Here's how the part is built. I have some questions about the finished solid (model axes, mm). Face numbers are marked on the shaded views. A direction names the side the tool comes from. Round coordinates to 2 decimals unless told otherwise and drop trailing zeros. Order: outer loops, then holes, each group sorted by start corner. A loop starts at its lowest first (then second) coordinate and runs counter-clockwise, first axis right, second up.
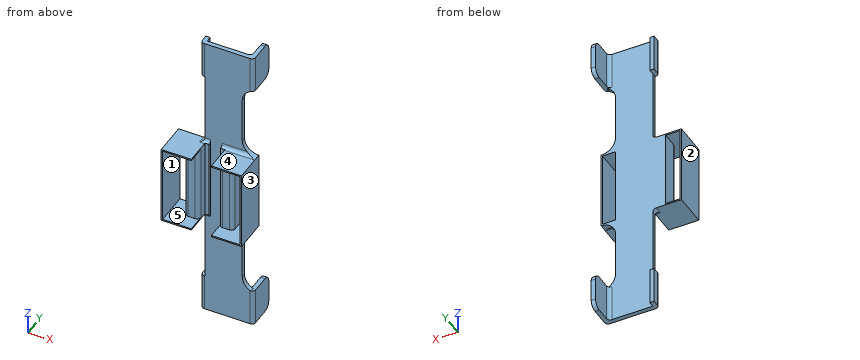
```python
from build123d import *

# Parameters (mm, degrees)
SKETCH1_W                 = 28
SKETCH1_H                 = 28
SKETCH1_W_2               = 27
SKETCH1_H_2               = 27
BOSS_EXTRUDE1_DEPTH       = 5
SKETCH2_W                 = 27
SKETCH2_H                 = 27
BOSS_EXTRUDE2_DEPTH       = 1
SKETCH4_W                 = 7
SKETCH4_H                 = 0.5
CUT_EXTRUDE1_DEPTH        = 4
CUT_EXTRUDE2_DEPTH        = 21.199009877
CUT_EXTRUDE2_DEPTH_BACK   = 21.199009877
SKETCH5_W                 = 5
SKETCH5_H                 = 27
SKETCH7_W                 = 5
SKETCH7_H                 = 27
BOSS_EXTRUDE3_DEPTH       = 4
BOSS_EXTRUDE4_DEPTH       = 5
BOSS_EXTRUDE5_DEPTH       = 5
SKETCH10_W                = 13
SKETCH10_H                = 105
BOSS_EXTRUDE6_DEPTH       = 1.5
SKETCH11_W                = 10
SKETCH11_H                = 28
SKETCH11_W_2              = 5
SKETCH11_H_2              = 27
BOSS_EXTRUDE7_DEPTH       = 1.5
SKETCH12_W                = 3
SKETCH12_H                = 13
BOSS_EXTRUDE8_DEPTH       = 1.5
SKETCH14_W                = 3
SKETCH14_H                = 13
BOSS_EXTRUDE9_DEPTH       = 1.5
FILLET1_R                 = 5
BOSS_EXTRUDE10_DEPTH      = 1
BOSS_EXTRUDE10_DEPTH_BACK = 0.5
SKETCH15_W                = 13
SKETCH15_H                = 10.000000066
FILLET2_R                 = 1.27
FILLET3_R                 = 1.27
FILLET4_R                 = 1.27
FILLET5_R                 = 1.27
SKETCH16_W                = 13
SKETCH16_H                = 3.5
BOSS_EXTRUDE11_DEPTH      = 1.5
FILLET6_R                 = 1.27
FILLET7_R                 = 1.27
FILLET8_R                 = 2.54
CUT_EXTRUDE3_DEPTH        = 1


with BuildPart() as part:
    # Sketch1 → Boss-Extrude1 (new body)
    with BuildSketch(Plane(origin=(0, 0, 0), x_dir=(1, 0, 0), z_dir=(0, 1, 0))):
        Rectangle(SKETCH1_W, SKETCH1_H)
        Rectangle(SKETCH1_W_2, SKETCH1_H_2, mode=Mode.SUBTRACT)
    extrude(amount=BOSS_EXTRUDE1_DEPTH)

    # Sketch4 → Cut-Extrude1 (cut)
    with BuildSketch(Plane.XZ):
        with Locations((0, 13.75)):
            Rectangle(SKETCH4_W, SKETCH4_H)
        with Locations((0, -13.75)):
            Rectangle(SKETCH4_W, SKETCH4_H)
    extrude(amount=-CUT_EXTRUDE1_DEPTH, mode=Mode.SUBTRACT)



with BuildPart() as body_2:
    # Sketch2 → Boss-Extrude2 (new body)
    with BuildSketch(Plane(origin=(0, 5, 0), x_dir=(1, 0, 0), z_dir=(0, 1, 0))):
        Rectangle(SKETCH2_W, SKETCH2_H)
    extrude(amount=-BOSS_EXTRUDE2_DEPTH)

    # Sketch5 → Cut-Extrude2 (cut, two sides: drawn at the far end of the back side and taken through both)
    with BuildSketch(Plane.XZ.offset(-4).offset(-CUT_EXTRUDE2_DEPTH_BACK)):
        with Locations((-11, 0)):
            Rectangle(SKETCH5_W, SKETCH5_H)
        with Locations((11, 0)):
            Rectangle(SKETCH5_W, SKETCH5_H)
    extrude(amount=CUT_EXTRUDE2_DEPTH + CUT_EXTRUDE2_DEPTH_BACK, mode=Mode.SUBTRACT)


with BuildPart() as part_1:
    add(part.part)

    add(body_2.part)  # Boss-Extrude3 merges body 2
    # Sketch7 → Boss-Extrude3 (add)
    with BuildSketch(Plane.XZ.offset(-4)):
        with Locations((-6, 0)):
            Rectangle(SKETCH7_W, SKETCH7_H)
        with Locations((6, 0)):
            Rectangle(SKETCH7_W, SKETCH7_H)
    extrude(amount=BOSS_EXTRUDE3_DEPTH)

    # Sketch8 → Boss-Extrude4 (add)
    with BuildSketch(Plane.XZ):
        Polygon((-13.5, -13.5), (-13.5, 13.5), (-3.5, 13.5), (-3.5, 14), (-14, 14), (-14, -14), (-3.5, -14), (-3.5, -13.5), align=None)
    extrude(amount=BOSS_EXTRUDE4_DEPTH)

    # Sketch9 → Boss-Extrude5 (add)
    with BuildSketch(Plane.XZ):
        Polygon((3.5, 14), (14, 14), (14, -14), (3.5, -14), (3.5, -13.5), (13.5, -13.5), (13.5, 13.5), (3.5, 13.5), align=None)
    extrude(amount=BOSS_EXTRUDE5_DEPTH)

    # Sketch10 → Boss-Extrude6 (add)
    with BuildSketch(Plane(origin=(0, 5, 0), x_dir=(1, 0, 0), z_dir=(0, 1, 0))):
        with Locations((2.5, 0)):
            Rectangle(SKETCH10_W, SKETCH10_H)
    extrude(amount=BOSS_EXTRUDE6_DEPTH)

    # Sketch11 → Boss-Extrude7 (add)
    # profile 1 of 2: a face of its own
    with BuildSketch(Plane(origin=(0, 5, 0), x_dir=(1, 0, 0), z_dir=(0, 1, 0))):
        with Locations((-9, 0)):
            Rectangle(SKETCH11_W, SKETCH11_H)
        with Locations((-11, 0)):
            Rectangle(SKETCH11_W_2, SKETCH11_H_2, mode=Mode.SUBTRACT)
    # profile 2 of 2: a face of its own
    with BuildSketch(Plane(origin=(0, 5, 0), x_dir=(1, 0, 0), z_dir=(0, 1, 0))):
        Polygon((9, 13.5), (9, 14), (14, 14), (14, -14), (9, -14), (9, -13.5), (13.5, -13.5), (13.5, 13.5), align=None)
    extrude(amount=BOSS_EXTRUDE7_DEPTH)

    # Sketch12 → Boss-Extrude8 (add)
    with BuildSketch(Plane(origin=(0, 6.5, 0), x_dir=(1, 0, 0), z_dir=(0, 1, 0))):
        with Locations((10.5, -46)):
            Rectangle(SKETCH12_W, SKETCH12_H)
    extrude(amount=-BOSS_EXTRUDE8_DEPTH)

    # Sketch14 → Boss-Extrude9 (add)
    with BuildSketch(Plane(origin=(0, 6.5, 0), x_dir=(1, 0, 0), z_dir=(0, 1, 0))):
        with Locations((10.5, 46)):
            Rectangle(SKETCH14_W, SKETCH14_H)
    extrude(amount=-BOSS_EXTRUDE9_DEPTH)

    # Fillet1
    # the kernel refuses this fillet: 5 mm, written as the material it adds along each edge
    with BuildSketch(Plane(origin=(9, 6.5, 39.5), x_dir=(0, 0, -1), z_dir=(0, -1, 0))) as fillet1_piece_1:
        with BuildLine():
            CenterArc((4.582575695, 5), FILLET1_R, 203.578178478, 66.421821522)
            Line((0, 3), (-0.091651514, 2.96))
            ThreePointArc((-0.091651514, 2.96), (-0.1, 1.5), (-0.1, 0))
            Line((-0.1, 0), (0, -0.1))
            Line((0, -0.1), (4.582575695, -0.1))
            Line((4.582575695, -0.1), (4.582575695, 0))
        make_face()
    extrude(amount=1.5)
    with BuildSketch(Plane(origin=(9, 5, 14), x_dir=(1, 0, 0), z_dir=(0, 1, 0))) as fillet1_piece_2:
        with BuildLine():
            CenterArc((FILLET1_R, -FILLET1_R), FILLET1_R, 90, 90)
            Line((0, -FILLET1_R), (-FILLET1_R * 0.02, -FILLET1_R))
            Line((-FILLET1_R * 0.02, -FILLET1_R), (-FILLET1_R * 0.02, FILLET1_R * 0.02))
            Line((-FILLET1_R * 0.02, FILLET1_R * 0.02), (FILLET1_R, FILLET1_R * 0.02))
            Line((FILLET1_R, FILLET1_R * 0.02), (FILLET1_R, 0))
        make_face()
    extrude(amount=1.5)
    with BuildSketch(Plane(origin=(9, 5, -14), x_dir=(1, 0, 0), z_dir=(0, 1, 0))) as fillet1_piece_3:
        with BuildLine():
            CenterArc((FILLET1_R, FILLET1_R), FILLET1_R, 180, 90)
            Line((0, FILLET1_R), (-FILLET1_R * 0.02, FILLET1_R))
            Line((-FILLET1_R * 0.02, FILLET1_R), (-FILLET1_R * 0.02, -FILLET1_R * 0.02))
            Line((-FILLET1_R * 0.02, -FILLET1_R * 0.02), (FILLET1_R, -FILLET1_R * 0.02))
            Line((FILLET1_R, -FILLET1_R * 0.02), (FILLET1_R, 0))
        make_face()
    extrude(amount=1.5)
    with BuildSketch(Plane(origin=(9, 6.5, -39.5), x_dir=(0, 0, 1), z_dir=(0, -1, 0))) as fillet1_piece_4:
        with BuildLine():
            CenterArc((4.582575695, -5), FILLET1_R, 90, 66.421821522)
            Line((0, -3), (-0.091651514, -2.96))
            ThreePointArc((-0.091651514, -2.96), (-0.1, -1.5), (-0.1, 0))
            Line((-0.1, 0), (0, 0.1))
            Line((0, 0.1), (4.582575695, 0.1))
            Line((4.582575695, 0.1), (4.582575695, 0))
        make_face()
    extrude(amount=1.5)

    # Sketch15 → Boss-Extrude10 (add, two sides: drawn at the far end of the back side and taken through both)
    with BuildSketch(Plane(origin=(12, 0, 0), x_dir=(0, 0, -1), z_dir=(1, 0, 0)).offset(-BOSS_EXTRUDE10_DEPTH_BACK)):
        with Locations((46, 10.000000033)):
            Rectangle(SKETCH15_W, SKETCH15_H)
        with Locations((-46, 10.000000033)):
            Rectangle(SKETCH15_W, SKETCH15_H)
    extrude(amount=BOSS_EXTRUDE10_DEPTH + BOSS_EXTRUDE10_DEPTH_BACK)

    # Fillet2
    fillet2_edges = [part_1.edges().sort_by_distance(p)[0] for p in [
        (11.5, 6.5, -46),
        (11.5, 6.5, 46),
    ]]
    fillet(fillet2_edges, radius=FILLET2_R)

    # Fillet3
    # the kernel refuses this fillet: 1.27 mm, written as the material it adds along each edge
    with BuildSketch(Plane(origin=(-4, 5, 14), x_dir=(0, 0, 1), z_dir=(1, 0, 0))) as fillet3_piece_1_section:
        with BuildLine():
            CenterArc((FILLET3_R, FILLET3_R), FILLET3_R, 180, 90)
            Line((0, FILLET3_R), (0, 0))
            Line((0, 0), (FILLET3_R, 0))
        make_face()
    fillet3_piece_1 = extrude(amount=18, mode=Mode.PRIVATE)
    fillet3_piece_1 = fillet3_piece_1 - Plane(origin=(14, 4.722255872, 19), x_dir=(1, 0, 0), z_dir=(0, -1, 0)) * Cylinder(5, 42, mode=Mode.PRIVATE)
    fillet3_piece_1 = split(fillet3_piece_1, bisect_by=Plane(origin=(-3.75, 4, 14.285759195), z_dir=(0, 1, 0)), keep=Keep.TOP, mode=Mode.PRIVATE)
    add(fillet3_piece_1)
    with BuildSketch(Plane(origin=(-4, 5, 14), x_dir=(0, 0, 1), z_dir=(1, 0, 0))) as fillet3_piece_2_section:
        with BuildLine():
            CenterArc((FILLET3_R, FILLET3_R), FILLET3_R, 180, 90)
            Line((0, FILLET3_R), (0, 0))
            Line((0, 0), (FILLET3_R, 0))
        make_face()
    fillet3_piece_2 = extrude(amount=21.175, mode=Mode.PRIVATE)
    fillet3_piece_2 = split(fillet3_piece_2, bisect_by=Plane(origin=(-3.5, 3.932655267, 14.008692454), z_dir=(-1, 0, 0)), keep=Keep.TOP, mode=Mode.PRIVATE)
    add(fillet3_piece_2)
    with BuildSketch(Plane(origin=(-7.175, 5, 14), x_dir=(0, 0, 1), z_dir=(1, 0, 0))) as fillet3_piece_3_section:
        with BuildLine():
            CenterArc((FILLET3_R, FILLET3_R), FILLET3_R, 180, 90)
            Line((0, FILLET3_R), (0, 0))
            Line((0, 0), (FILLET3_R, 0))
        make_face()
    fillet3_piece_3 = extrude(amount=21.175, mode=Mode.PRIVATE)
    fillet3_piece_3 = fillet3_piece_3 - Plane(origin=(14, 3.932300045, 19), x_dir=(1, 0, 0), z_dir=(0, -1, 0)) * Cylinder(5, 48, mode=Mode.PRIVATE)
    fillet3_piece_3 = split(fillet3_piece_3, bisect_by=Plane(origin=(3.5, 3.932300045, 14.008616185), z_dir=(1, 0, 0)), keep=Keep.TOP, mode=Mode.PRIVATE)
    add(fillet3_piece_3)
    with BuildSketch(Plane(origin=(14, 5, -14), x_dir=(0, 0, -1), z_dir=(-1, 0, 0))) as fillet3_piece_4_section:
        with BuildLine():
            CenterArc((FILLET3_R, FILLET3_R), FILLET3_R, 180, 90)
            Line((0, FILLET3_R), (0, 0))
            Line((0, 0), (FILLET3_R, 0))
        make_face()
    fillet3_piece_4 = extrude(amount=18, mode=Mode.PRIVATE)
    fillet3_piece_4 = fillet3_piece_4 - Plane(origin=(14, 4.711484111, -19), x_dir=(1, 0, 0), z_dir=(0, -1, 0)) * Cylinder(5, 42, mode=Mode.PRIVATE)
    fillet3_piece_4 = split(fillet3_piece_4, bisect_by=Plane(origin=(8.027122346, 4, -14.26821747), z_dir=(0, 1, 0)), keep=Keep.TOP, mode=Mode.PRIVATE)
    add(fillet3_piece_4)
    with BuildSketch(Plane(origin=(14, 5, -14), x_dir=(0, 0, -1), z_dir=(-1, 0, 0))) as fillet3_piece_5_section:
        with BuildLine():
            CenterArc((FILLET3_R, FILLET3_R), FILLET3_R, 180, 90)
            Line((0, FILLET3_R), (0, 0))
            Line((0, 0), (FILLET3_R, 0))
        make_face()
    fillet3_piece_5 = extrude(amount=21.175, mode=Mode.PRIVATE)
    fillet3_piece_5 = fillet3_piece_5 - Plane(origin=(14, 3.932300045, -19), x_dir=(1, 0, 0), z_dir=(0, -1, 0)) * Cylinder(5, 48, mode=Mode.PRIVATE)
    fillet3_piece_5 = split(fillet3_piece_5, bisect_by=Plane(origin=(3.5, 3.932300045, -14.008616185), z_dir=(1, 0, 0)), keep=Keep.TOP, mode=Mode.PRIVATE)
    add(fillet3_piece_5)
    with BuildSketch(Plane(origin=(17.175, 5, -14), x_dir=(0, 0, -1), z_dir=(-1, 0, 0))) as fillet3_piece_6_section:
        with BuildLine():
            CenterArc((FILLET3_R, FILLET3_R), FILLET3_R, 180, 90)
            Line((0, FILLET3_R), (0, 0))
            Line((0, 0), (FILLET3_R, 0))
        make_face()
    fillet3_piece_6 = extrude(amount=21.175, mode=Mode.PRIVATE)
    fillet3_piece_6 = split(fillet3_piece_6, bisect_by=Plane(origin=(-3.5, 3.932655267, -14.008692454), z_dir=(-1, 0, 0)), keep=Keep.TOP, mode=Mode.PRIVATE)
    add(fillet3_piece_6)

    # Fillet4
    fillet4_edges = [part_1.edges().sort_by_distance(p)[0] for p in [
        (-3.5, 0, 0),
        (3.5, 0, 0),
        (-8.5, 0, 0),
        (8.5, 0, 0),
    ]]
    fillet(fillet4_edges, radius=FILLET4_R)

    # Fillet5
    fillet5_edges = [part_1.edges().sort_by_distance(p)[0] for p in [
        (-4, 5.115, -14),
        (-4, 5.115, 14),
    ]]
    fillet(fillet5_edges, radius=FILLET5_R)

    # Sketch16 → Boss-Extrude11 (add)
    with BuildSketch(Plane.ZY.offset(4)):
        with Locations((-46, 6.75)):
            Rectangle(SKETCH16_W, SKETCH16_H)
        with Locations((46, 6.75)):
            Rectangle(SKETCH16_W, SKETCH16_H)
    extrude(amount=BOSS_EXTRUDE11_DEPTH)

    # Fillet6
    fillet6_edges = [part_1.edges().sort_by_distance(p)[0] for p in [
        (-5.5, 5, 46),
        (-5.5, 5, -46),
    ]]
    fillet(fillet6_edges, radius=FILLET6_R)

    # Fillet7
    fillet7_edges = [part_1.edges().sort_by_distance(p)[0] for p in [
        (13, 5, 46),
        (13, 5, -46),
    ]]
    fillet(fillet7_edges, radius=FILLET7_R)

    # Fillet8
    fillet8_edges = [part_1.edges().sort_by_distance(p)[0] for p in [
        (12.25, 15.000000066, -52.5),
        (12.25, 15.000000066, -39.5),
        (12.25, 15.000000066, 39.5),
        (12.25, 15.000000066, 52.5),
    ]]
    fillet(fillet8_edges, radius=FILLET8_R)

    # Sketch17 → Cut-Extrude3 (cut)
    with BuildSketch(Plane.XZ.offset(-4)):
        Polygon((-2, 14.029032635), (-2, -14.029032635), (-2, -17.474025738), (2, -17.474025738), (2, -14.029032635), (2, 14.029032635), (2, 17.175749071), (-2, 17.175749071), align=None)
    extrude(amount=-CUT_EXTRUDE3_DEPTH, mode=Mode.SUBTRACT)


solid = part_1.part
```
1. On a 3-axis mill with a long thin cutter (end or side, diameter ignored), from which of +Z, -Z, +X, -X, +Y, -Y can I reach the whole of each face in a straight line? I mean the marked faces 4 and 5. Say none if no direction works.
Evaluation:
face 4: +Z, +X, -X, -Y
face 5: -Y
2. If we section it at A-A, the plane z = 5: Write out the boundary of the cut face in (x, y), and give its area (3 significant figures).
Evaluation:
outline: (-14, -5) - (-13.5, -5) - (-13.5, 6.5) - (-14, 6.5) - close; (-8.5, 1.27) arc R1.27 ccw to (-7.23, 0) - (-4.77, 0) arc R1.27 ccw to (-3.5, 1.27) - (-3.5, 4) - (-2, 4) - (-2, 5) - (2, 5) - (2, 4) - (3.5, 4) - (3.5, 1.27) arc R1.27 ccw to (4.77, 0) - (7.23, 0) arc R1.27 ccw to (8.5, 1.27) - (8.5, 5) - (9, 5) - (9, 6.5) - (-8.5, 6.5) - close; (13.5, -5) - (14, -5) - (14, 6.5) - (13.5, 6.5) - close
area: 89.4 mm2
3. I need wall thicknesses on probe 1 along X at (y, z) = (2, -5); probe 2 along Z at (x, y) = (-9, -0.5). Which ranges of each line are inside material? Lowest first, please.
Evaluation:
probe 1: x = -14 to -13.5, -8.5 to -3.5, 3.5 to 8.5, 13.5 to 14
probe 2: z = -14 to -13.5, 13.5 to 14
4. If we section it at B-B, the plane x = -11: Write out the boundary of the cut face in (y, z), and give its area (3 significant figures).
Evaluation:
outline: (-5, -14) - (6.5, -14) - (6.5, -13.5) - (-5, -13.5) - close; (-5, 13.5) - (6.5, 13.5) - (6.5, 14) - (-5, 14) - close
area: 11.5 mm2
5. If we section it at D-D, the plane y = 2.25: Write out the boundary of the cut face in (x, z).
Evaluation:
outline: (-14, -14) - (-3.5, -14) - (-3.5, 14) - (-14, 14) - close; (3.5, -14) - (14, -14) - (14, 14) - (3.5, 14) - close; hole (-13.5, -13.5) - (-8.5, -13.5) - (-8.5, 13.5) - (-13.5, 13.5) - close; hole (8.5, -13.5) - (13.5, -13.5) - (13.5, 13.5) - (8.5, 13.5) - close
6. If we mould it in two halves opening along X, with no side actions, what happens to the marked faces 1, 2 and 3? For each: released by +X, released by -X, zero draft, split by the parting line, or undercut.
Evaluation:
face 1: undercut
face 2: released by -X
face 3: released by +X
7. If we section it at C-C, the plane y = 10.5: Write out the boundary of the cut face in (x, z), and give its area (3 significant figures).
Evaluation:
outline: (11.5, -52.5) - (13, -52.5) - (13, -39.5) - (11.5, -39.5) - close; (11.5, 39.5) - (13, 39.5) - (13, 52.5) - (11.5, 52.5) - close
area: 39.0 mm2
8. I'm going to push flat-ended pins straight in: P1, Ø3, axis at x = -5, y = 1, coming from the -Z side; P2, Ø5, axis at x = 8.5, y = 0.5, coming from the +Z side; P3, Ø3, axis at x = 10, y = 3, coming from the +Z side. Where does each tip first touch, or does it pass through?
Evaluation:
P1: stops at z = -14
P2: stops at z = 14
P3: stops at z = 14.26
